The listing builds one solid part. Answer for the finished solid, in the listing's coordinates (mm). Face numbers are marked on the shaded views. A direction names the side the tool comes from. Coordinates: 2 decimals unless noted, no trailing zeros. Write each loop counter-clockwise with the first axis right and the second up, starting at its lowest first coordinate (ties: lowest second). Pieces come first, ordered by that corner, then holes.
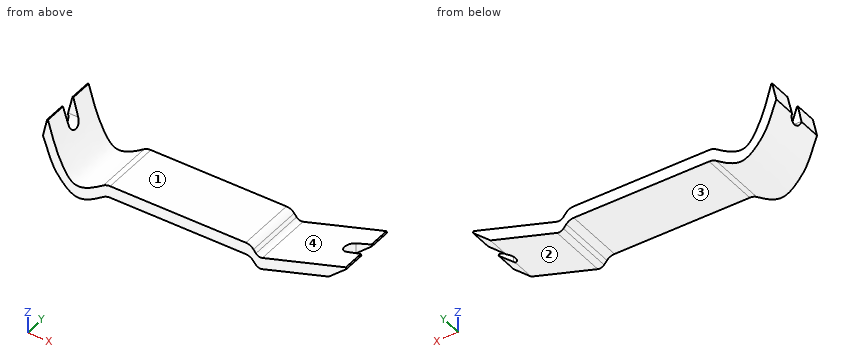
from build123d import *

# Parameters (mm, degrees)
F1_DEPTH = 30
F3_START = -60
F3_DEPTH = 20
F5_DEPTH = 15


with BuildPart() as f1:
    # F0 (on Front) → F1 (new body)
    with BuildSketch(Plane.XZ):
        with BuildLine():
            Line((-73.2672911175, 26.5288166702), (-75.3194466233, 17.3055510968))
            add(Edge.make_bspline(
                [(-75.3194466233, 17.3055510968), (-70.9649776781, 4.4868251649), (-69.3683816602, 1.5297526715), (-58.7741680812, -10.797200258), (-50.064963712, -5.329070788), (-44.9501895242, -1.7400602878)],
                knots=[0, 0, 0, 0, 0.374435083, 0.6549537817, 0.9687940857, 0.9687940857, 0.9687940857, 0.9687940857], degree=3))
            ThreePointArc((-44.9501895242, -1.7400602878), (-43.310919022, -0.9301366905), (-41.5038310897, -0.6515380228))
            Line((-41.5038310897, -0.6515380228), (26.6625816426, -0.6515380228))
            ThreePointArc((26.6625816426, -0.6515380228), (28.7383095769, -1.1027630731), (30.4393893345, -2.3749966056))
            Line((30.4393893345, -2.3749966056), (31.9053379066, -4.0647679645))
            ThreePointArc((31.9053379066, -4.0647679645), (33.3557980505, -4.9858409878), (35.0738020651, -4.9599112993))
            Line((35.0738020651, -4.9599112993), (68.6204453138, 5.6206840096))
            Line((68.6204453138, 5.6206840096), (77.4316421282, 13.3455851134))
            Line((77.4316421282, 13.3455851134), (77.1660596132, 14.18763621))
            Line((77.1660596132, 14.18763621), (35.1581896409, 0.9383740209))
            ThreePointArc((35.1581896409, 0.9383740209), (33.3767909305, 0.9311107565), (31.9053377109, 1.9352320355))
            Line((31.9053377109, 1.9352320355), (30.6995972244, 3.4554789281))
            ThreePointArc((30.6995972244, 3.4554789281), (28.9575644986, 4.8504107083), (26.7821432468, 5.3484619772))
            Line((26.7821432468, 5.3484619772), (-41.5150223961, 5.3484619772))
            ThreePointArc((-41.5150223961, 5.3484619772), (-43.3039602481, 5.0755643302), (-44.9301657899, 4.2816957645))
            add(Edge.make_bspline(
                [(-72.8339403868, 26.5288166702), (-69.6615353227, 15.0968804955), (-66.54271386, 6.9837829262), (-59.2191643212, -4.6015653314), (-50.1028643922, 0.7007774012), (-44.9301657899, 4.2816957645)],
                knots=[0, 0, 0, 0, 0.3985404471, 0.6568286308, 0.9694419113, 0.9694419113, 0.9694419113, 0.9694419113], degree=3))
            Line((-72.8339403868, 26.5288166702), (-73.2672911175, 26.5288166702))
        make_face()
    extrude(amount=F1_DEPTH)

    # F2 (on Right) → F3 (cut)
    with BuildSketch(Plane.YZ.offset(F3_START)):
        with BuildLine():
            ThreePointArc((-18.5974218494, 17.528353259), (-15.0974218494, 14.028353259), (-11.5974218494, 17.528353259))
            Line((-11.5974218494, 17.528353259), (-11.2484100663, 26.7637830809))
            Line((-11.2484100663, 26.7637830809), (-18.946434269, 26.7637830809))
            Line((-18.946434269, 26.7637830809), (-18.5974218494, 17.528353259))
        make_face()
    extrude(amount=-F3_DEPTH, mode=Mode.SUBTRACT)

    # F4 (on Top) → F5 (cut)
    with BuildSketch(Plane.XY):
        with BuildLine():
            Line((78.2688707113, -11.0539328307), (69.7815798237, -11.5))
            ThreePointArc((69.7815798237, -11.5), (66.2815798237, -15), (69.7815798237, -18.5))
            Line((69.7815798237, -18.5), (78.2688707113, -18.9460671693))
            Line((78.2688707113, -18.9460671693), (78.2688707113, -11.0539328307))
        make_face()
    extrude(amount=F5_DEPTH, mode=Mode.SUBTRACT)


solid = f1.part
1. A tool of negligible diameter and unlimited length cuts with its end or side. For the marked faces 3 and 4, from which of +Z, -Z, +X, -X, +Y, -Y can it reach the whole face along a straight path? Write none if from no direction.
Results found:
face 3: -Z, +Y, -Y
face 4: +Z, +Y, -Y
2. Section A-A on x = -15 is taken. Give the vertices of the cut face in (y, z).
Results found:
outline: (-30, -0.65) - (0, -0.65) - (0, 5.35) - (-30, 5.35) - close
3. Find the intervals of material crossed by L1, parallel to Z at x = 6.5, y = -14.5; L2, parallel to Z at x = -49.5, y = -26; L3, parallel to X at y = -2.5, z = 17, in increasing order.
Results found:
L1: z = -0.65 to 5.35
L2: z = -4.76 to 1.32
L3: x = -75.22 to -70.01
4. Flat-ended cylindrical pins translate along their axes: P1, Ø1, axis at y = -17.5, z = 5.5, coming from the +X side; P2, Ø5, axis at y = -6, z = 18.5, coming from the +X side; P3, Ø2, axis at x = -12.5, y = -26.5, coming from the +Z side; P4, Ø10, axis at x = 37.5, z = 12, coming from the +Y side. Find the tip coordinate at first contact, or state that the pin passes through.
Results found:
P1: stops at x = 67.98
P2: stops at x = -69.68
P3: stops at z = 5.35
P4: passes through
5. For a pull along X with two mould halves and no side action, classify the marked faces 1 and 2 as pulls with the +X half, pulls with the -X half, needs draft (parallel to the pull), parting line crosses it, or undercut.
Results found:
face 1: undercut
face 2: pulls with the +X half
